```python
from build123d import *

# Parameters (mm, degrees)
SKETCH_1_W          = 17.8
SKETCH_1_H          = 42.8
EXTRUDE_1_DEPTH     = 5.5
SKETCH_6_R          = 2.15
CUT_EXTRUDE_3_DEPTH = 10
CUT_EXTRUDE_4_DEPTH = 3
SKETCH_10_R         = 6
EXTRUDE_5_DEPTH     = 18.8
SKETCH_12_W         = 9.298485121
SKETCH_12_H         = 14.239097106
CUT_EXTRUDE_5_DEPTH = 12
SKETCH_13_W         = 8.310362724
SKETCH_13_H         = 15.683275995
CUT_EXTRUDE_6_DEPTH = 12
SKETCH_14_R         = 3
CUT_EXTRUDE_7_DEPTH = 22


with BuildPart() as part:
    # 草图1 → 凸台-拉伸1 (new body)
    with BuildSketch(Plane(origin=(0, 0, 0), x_dir=(1, 0, 0), z_dir=(0, 1, 0))):
        with Locations((8.9, -21.4)):
            Rectangle(SKETCH_1_W, SKETCH_1_H)
    extrude(amount=EXTRUDE_1_DEPTH)

    # 草图6 → 切除-拉伸3 (cut)
    with BuildSketch(Plane(origin=(0, 5.5, 0), x_dir=(1, 0, 0), z_dir=(0, 1, 0))):
        with Locations(Location((5.420411498, -5.65, 0), (0, 0, 270))):
            Circle(SKETCH_6_R)
        with Locations(Location((5.420411498, -37.15, 0), (0, 0, 270))):
            Circle(SKETCH_6_R)
    extrude(amount=-CUT_EXTRUDE_3_DEPTH, mode=Mode.SUBTRACT)

    # 草图7 → 切除-拉伸4 (cut)
    with BuildSketch(Plane(origin=(0, 5.5, 0), x_dir=(1, 0, 0), z_dir=(0, 1, 0))):
        Polygon((2.920411498, -1.319872981), (7.920411498, -1.319872981), (10.420411498, -5.65), (7.920411498, -9.980127019), (2.920411498, -9.980127019), (0.420411498, -5.65), align=None)
        Polygon((0.420411498, -37.15), (2.920411498, -32.819872981), (7.920411498, -32.819872981), (10.420411498, -37.15), (7.920411498, -41.480127019), (2.920411498, -41.480127019), align=None)
    extrude(amount=-CUT_EXTRUDE_4_DEPTH, mode=Mode.SUBTRACT)

    # 草图10 → 凸台-拉伸5 (add)
    with BuildSketch(Plane.XY.offset(30.8)):
        with Locations((17.8, 2.75)):
            Circle(SKETCH_10_R)
    extrude(amount=-EXTRUDE_5_DEPTH)

    # 草图12 → 切除-拉伸5 (cut)
    with BuildSketch(Plane.XY.offset(42.8)):
        with Locations((15.774868429, 2.737331764)):
            Rectangle(SKETCH_12_W, SKETCH_12_H)
    extrude(amount=-CUT_EXTRUDE_5_DEPTH, mode=Mode.SUBTRACT)

    # 草图13 → 切除-拉伸6 (cut)
    with BuildSketch(Plane(origin=(0, 0, 0), x_dir=(-1, 0, 0), z_dir=(0, 0, -1))):
        with Locations((-15.838209607, 3.510094151)):
            Rectangle(SKETCH_13_W, SKETCH_13_H)
    extrude(amount=-CUT_EXTRUDE_6_DEPTH, mode=Mode.SUBTRACT)

    # 草图14 → 切除-拉伸7 (cut)
    with BuildSketch(Plane.XY.offset(30.8)):
        with Locations((17.8, 2.75)):
            Circle(SKETCH_14_R)
    extrude(amount=-CUT_EXTRUDE_7_DEPTH, mode=Mode.SUBTRACT)


solid = part.part
```
Here's how the part is built. I have some questions about the finished solid (model axes, mm). A direction names the side the tool comes from. Coordinates: 2 decimals unless noted, no trailing zeros. Write each loop counter-clockwise with the first axis right and the second up, starting at its lowest first coordinate (ties: lowest second). Pieces come first, ordered by that corner, then holes. Notation, with made-up numbers: (25, 35.25) -> (42, 35.25) arc R18 cw to (42, 48.25) -> close; hole circle Ø5 at (68.5, -0.75). An arc over 180 degrees is marked (long way). Use a Markdown table: item, result. Add a question column.
(1) If we section it at B-B, the plane y = 4.5: Write out the boundary of the cut face in (x, z), and give its area (3 significant figures).
(2) If we section it at C-C, the plane z = 36: Write out the boundary of the cut face in (x, y), and give its area (3 significant figures).
(3) I'm going to push flat-ended pins straight in: P1, Ø2.5, axis at x = 5.42, z = 5.65, coming from the +Y side; P2, Ø6, axis at x = 9, z = 12, coming from the +Y side; P3, Ø6, axis at x = 19, y = 0, coming from the +Z side; P4, Ø6, axis at x = 19, y = 2.5, coming from the -Z side. Where does each tip first touch, or does it pass through?
(4) If we section it at D-D, the plane z = 14.5: Write out the boundary of the cut face in (x, y).
(5) Please list where these lines run through material, in increasing order: line 1 (Z direction, x = 4, y = 4.25); line 2 (X direction, y = 0.65, z = 37.15); line 3 (X direction, y = 1.4, z = 5.65).
(6) For faces 1 (the flat face through (3, 2.5, 37)), 2 (the flat face through (19, 6, 12)), 3 (the flat face through (6, 5.5, 21)), which set-ups out of +Z, -Z, +X, -X, +Y, -Y let a thin tool reach every point of the face, with its end or its side?
(7) If we section it at A-A, the plane x = 17.8: Write out the boundary of the cut face in (y, z), and give its area (3 significant figures).
(8) We'd pull the mould along Z, two halves only. Please class faces 4 (the flat face through (5, 4, 32.82)), 5 (the flat face through (14.6, 2.8, 30.8)), 6 (the flat face through (6, 3, 0)): +Z half, -Z half, draft (parallel to the pull), parting line (faces both ways), or undercut.
Outcome:
| question | item | result |
|---|---|---|
| 1 | outline | (0, 0) -> (11.68, 0) -> (11.68, 12) -> (15.36, 12) -> (15.36, 30.8) -> (11.13, 30.8) -> (11.13, 42.8) -> (0, 42.8) -> close; (20.24, 12) -> (23.54, 12) -> (23.54, 30.8) -> (20.24, 30.8) -> close; hole (0.42, 5.65) -> (2.92, 1.32) -> (7.92, 1.32) -> (10.42, 5.65) -> (7.92, 9.98) -> (2.92, 9.98) -> close; hole (0.42, 37.15) -> (2.92, 32.82) -> (7.92, 32.82) -> (10.42, 37.15) -> (7.92, 41.48) -> (2.92, 41.48) -> close |
| 1 | area | 495 mm^2 |
| 2 | outline | (0, 0) -> (3.6, 0) -> (3.6, 2.5) -> (1.08, 2.5) -> (1.08, 5.5) -> (0, 5.5) -> close; (7.24, 0) -> (11.13, 0) -> (11.13, 5.5) -> (9.76, 5.5) -> (9.76, 2.5) -> (7.24, 2.5) -> close |
| 2 | area | 26.1 mm^2 |
| 3 | P1 | passes through |
| 3 | P2 | stops at y = 5.5 |
| 3 | P3 | stops at z = 30.8 |
| 3 | P4 | stops at z = 12 |
| 4 | outline | (0, 0) -> (12.47, 0) arc R6 ccw (long way) to (12.47, 5.5) -> (0, 5.5) -> close; hole circle Ø6 at (17.8, 2.75) |
| 5 | line 1 | z = 0 to 1.32, 9.98 to 32.82, 41.48 to 42.8 |
| 5 | line 2 | x = 0 to 3.27, 7.57 to 11.13 |
| 5 | line 3 | x = 0 to 3.27, 7.57 to 11.68 |
| 6 | face 1 | +Y |
| 6 | face 2 | -Z, +X, +Y, -Y |
| 6 | face 3 | +Z, -Z, -X, +Y |
| 7 | outline | (-3.25, 12) -> (-0.25, 12) -> (-0.25, 30.8) -> (-3.25, 30.8) -> close; (5.75, 12) -> (8.75, 12) -> (8.75, 30.8) -> (5.75, 30.8) -> close |
| 7 | area | 113 mm^2 |
| 8 | face 4 | undercut |
| 8 | face 5 | +Z half |
| 8 | face 6 | -Z half |
